Read the model definition and answer for the solid it produces. Units are mm, in the model's axes. A direction names the side the tool comes from. Coordinates: 2 decimals unless noted, no trailing zeros. Loops run counter-clockwise (first coordinate to the right, second up) from the corner with the lowest first, then second, coordinate; pieces in that order, holes last.
Q1. Which of the six approach directions +Z, -Z, +X, -X, +Y, -Y give full straight-line access (tool end or side, diameter ignored) to faces 1 (the face through (-22.5, -8.6, 5.4)), 2 (the face through (-12.893, -35.876, 10.114))?
Q2. Section A-A (y = -20) is taken. Give the vertices of the cut face in (x, z), then the cut area to 3 significant figures.
Q3. Flat-ended cylindrical pins translate along their axes: P1, Ø8, axis at x = -20, z = 5.5, coming from the +Y side; P2, Ø1.5, axis at x = 19, z = 5, coming from the +Y side; P3, Ø3, axis at x = -19, y = -20, coming from the -Z side. Find the tip coordinate at first contact, or state that the pin passes through.
Q4. Straight lines are drawn through the part: line 1 (Z direction, x = -20, y = -12.5); line 2 (Z direction, x = -21, y = -11); line 3 (Y direction, x = 11.5, z = 11.5). For each, find the intervals that lie inside material, in ascending order.
Q5. Section B-B (z = 25.5) is taken. Give the vertices of the cut face in (x, y).
Q6. Section C-C (y = -2.5) is taken. Give the vertices of the cut face in (x, z), then the cut area to 3 significant figures.
Q7. Section D-D (x = 0) is taken. Give the vertices of the cut face in (y, z), then the cut area to 3 significant figures.
Q8. The mould has two halves that part along X. Classify faces 3 (the face through (16, -40, 17)), 4 (the face through (13.977, -35.876, 10.114)), 5 (the face through (24, -20, 17)): pulls with the +X half, pulls with the -X half, needs draft (parallel to the pull), parting line crosses it, or undercut.
from build123d import *

# Parameters (mm, degrees)
BOSS_EXTRUDE1_DEPTH = 35
CHAMFER2_SIZE       = 0.3
SKETCH2_R           = 2.5
CUT_EXTRUDE1_DEPTH  = 17
SKETCH3_R           = 2.5
CUT_EXTRUDE2_DEPTH  = 20
CHAMFER3_SIZE       = 0.5


with BuildPart() as part:
    # Sketch1 → Boss-Extrude1 (new body)
    with BuildSketch(Plane.XY):
        with BuildLine():
            Line((24, 0), (-24, 0))
            Line((-24, 0), (-24, -40))
            Line((-24, -40), (-8.5, -40))
            Line((-8.5, -40), (-8.5, -31.187157816))
            ThreePointArc((-8.5, -31.187157816), (0, -5.95), (8.5, -31.187157816))
            Line((8.5, -31.187157816), (8.5, -40))
            Line((8.5, -40), (24, -40))
            Line((24, -40), (24, 0))
        make_face()
    extrude(amount=BOSS_EXTRUDE1_DEPTH)

    # Chamfer2
    chamfer2_edges = [part.edges().sort_by_distance(p)[0] for p in [
        (0, -5.95, 35),
        (-8.5, -35.593578908, 0),
        (-16.25, -40, 0),
        (8.5, -35.593578908, 35),
        (-24, -40, 17.5),
        (-24, 0, 17.5),
        (24, 0, 17.5),
        (24, -40, 17.5),
        (8.5, -40, 17.5),
        (-8.5, -40, 17.5),
        (16.25, -40, 35),
        (24, -20, 35),
        (0, 0, 35),
        (-24, -20, 35),
        (-16.25, -40, 35),
        (-8.5, -35.593578908, 35),
        (-24, -20, 0),
        (0, 0, 0),
        (24, -20, 0),
        (16.25, -40, 0),
        (8.5, -35.593578908, 0),
        (0, -5.95, 0),
    ]]
    chamfer(chamfer2_edges, length=CHAMFER2_SIZE)

    # Sketch2 → Cut-Extrude1 (cut)
    with BuildSketch(Plane(origin=(0, 0, 0), x_dir=(1, 0, 0), z_dir=(0, 1, 0))):
        with Locations((-20, -5.5)):
            Circle(SKETCH2_R)
        with Locations((20, -5.5)):
            Circle(SKETCH2_R)
        with Locations((20, -29.5)):
            Circle(SKETCH2_R)
        with Locations((-20, -29.5)):
            Circle(SKETCH2_R)
    extrude(amount=-CUT_EXTRUDE1_DEPTH, mode=Mode.SUBTRACT)

    # Sketch3 → Cut-Extrude2 (cut)
    with BuildSketch(Plane(origin=(0, 0, 0), x_dir=(-1, 0, 0), z_dir=(0, 0, -1))):
        with Locations((-13.435028843, -33.435028843)):
            Circle(SKETCH3_R)
        with Locations((13.435028843, -33.435028843)):
            Circle(SKETCH3_R)
        with Locations((13.435028843, -6.564971157)):
            Circle(SKETCH3_R)
        with Locations((-13.435028843, -6.564971157)):
            Circle(SKETCH3_R)
        with Locations((-19, -20)):
            Circle(SKETCH3_R)
        with Locations((19, -20)):
            Circle(SKETCH3_R)
    extrude(amount=-CUT_EXTRUDE2_DEPTH, mode=Mode.SUBTRACT)

    # Chamfer3
    chamfer3_edges = [part.edges().sort_by_distance(p)[0] for p in [
        (17.5, 0, 29.5),
        (-22.5, 0, 29.5),
        (15.935028843, -33.435028843, 0),
        (-10.935028843, -33.435028843, 0),
        (-10.935028843, -6.564971157, 0),
        (-16.5, -20, 0),
        (21.5, -20, 0),
        (-22.5, 0, 5.5),
        (17.5, 0, 5.5),
    ]]
    chamfer(chamfer3_edges, length=CHAMFER3_SIZE)


solid = part.part
Numbers:
1. face 1: +Y
1. face 2: -Z
2. outline: (-24, 0.3) - (-23.7, 0) - (-22, 0) - (-21.5, 0.5) - (-21.5, 20) - (-16.5, 20) - (-16.5, 0.5) - (-16, 0) - (-14.35, 0) - (-14.05, 0.3) - (-14.05, 34.7) - (-14.35, 35) - (-23.7, 35) - (-24, 34.7) - close; (14.05, 0.3) - (14.35, 0) - (16, 0) - (16.5, 0.5) - (16.5, 20) - (21.5, 20) - (21.5, 0.5) - (22, 0) - (23.7, 0) - (24, 0.3) - (24, 34.7) - (23.7, 35) - (14.35, 35) - (14.05, 34.7) - close
2. area: 496 mm2
3. P1: stops at y = 0
3. P2: stops at y = -17
3. P3: stops at z = 20
4. line 1: z = 0 to 3, 8 to 27, 32 to 35
4. line 2: z = 0 to 3.21, 7.79 to 27.21, 31.79 to 35
4. line 3: y = -40 to -35.02, -31.85 to -28.07, -11.93 to -8.15, -4.98 to 0
5. outline: (-24, -39.7) - (-23.7, -40) - (-8.8, -40) - (-8.5, -39.7) - (-8.5, -31.19) arc R14.05 cw (long way) to (8.5, -31.19) - (8.5, -39.7) - (8.8, -40) - (23.7, -40) - (24, -39.7) - (24, -0.3) - (23.7, 0) - (-23.7, 0) - (-24, -0.3) - close
6. outline: (-24, 0.3) - (-23.7, 0) - (23.7, 0) - (24, 0.3) - (24, 34.7) - (23.7, 35) - (-23.7, 35) - (-24, 34.7) - close; hole circle Ø5 at (-20, 5.5); hole circle Ø5 at (-20, 29.5); hole circle Ø5 at (20, 5.5); hole circle Ø5 at (20, 29.5)
6. area: 1,600 mm2
7. outline: (-5.95, 0.3) - (-5.65, 0) - (-0.3, 0) - (0, 0.3) - (0, 34.7) - (-0.3, 35) - (-5.65, 35) - (-5.95, 34.7) - close
7. area: 208 mm2
8. face 3: needs draft
8. face 4: undercut
8. face 5: pulls with the +X half
